```python
from build123d import *

# Parameters (mm, degrees)
SKETCH_5_R               = 3.5
EXTRUDE_2_DEPTH          = 13
SKETCH_6_R               = 3
CUT_EXTRUDE_2_DEPTH      = 13
CUT_EXTRUDE_2_DEPTH_BACK = 13
SKETCH_7_R               = 4.5
EXTRUDE_3_DEPTH          = 1.5


with BuildPart() as part:
    # Sketch 1 → Revolve 5 (revolve)
    with BuildSketch(Plane(origin=(0, 0, 0), x_dir=(1, 0, 0), z_dir=(0, 1, 0))):
        with BuildLine():
            Line((0, 5), (0, -5))
            ThreePointArc((0, -5), (-5, 0), (0, 5))
        make_face()
    revolve(axis=Axis((0, 0, -5), (0, 0, 1)))

    # Sketch 5 → Extrude 2 (add)
    with BuildSketch(Plane.XY):
        Circle(SKETCH_5_R)
    extrude(amount=EXTRUDE_2_DEPTH)

    # Sketch 6 → Cut-Extrude 2 (cut, two sides)
    with BuildSketch(Plane(origin=(0, 0, 0), x_dir=(0, 0, -1), z_dir=(1, 0, 0))) as cut_extrude_2_sk:
        Circle(SKETCH_6_R)
    extrude(amount=CUT_EXTRUDE_2_DEPTH, mode=Mode.SUBTRACT)
    extrude(cut_extrude_2_sk.sketch, amount=-CUT_EXTRUDE_2_DEPTH_BACK, mode=Mode.SUBTRACT)

    # Sketch 7 → Extrude 3 (add)
    with BuildSketch(Plane.XY.offset(5)):
        Circle(SKETCH_7_R)
    extrude(amount=-EXTRUDE_3_DEPTH)


solid = part.part
```
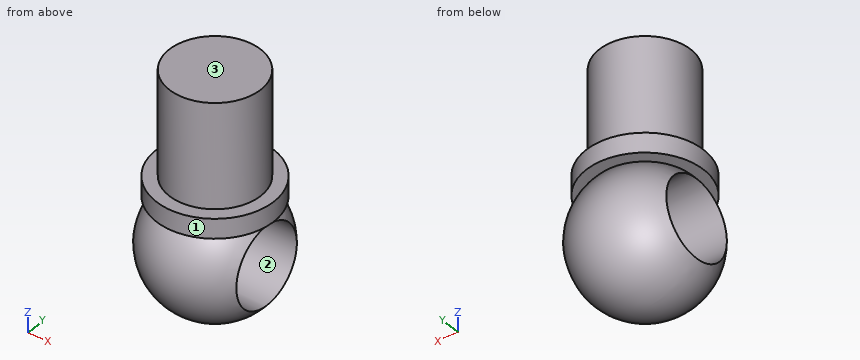
The listing builds one solid part. Answer for the finished solid, in the listing's coordinates (mm). Face numbers are marked on the shaded views. Round coordinates to 2 decimals unless told otherwise and drop trailing zeros. Write each loop counter-clockwise with the first axis right and the second up, starting at its lowest first coordinate (ties: lowest second). Pieces come first, ordered by that corner, then holes. Notation, with made-up numbers: (17, -5) -> (50, -5) arc R21 ccw to (50, 6) -> close; hole circle Ø6 at (46.5, 80.25). An arc over 180 degrees is marked (long way). Use CSV: the item, a comma, the result in double quotes. Start each with the question number.
(1) Section B-B on x = 0 is taken. Give the vertices of the cut face in (y, z).
(2) Section D-D on y = -2.75 is taken. Give the vertices of the cut face in (x, z), then the cut area to 3 significant figures.
(3) Section C-C on z = 0 is taken. Give the vertices of the cut face in (x, y).
(4) Each of these flat-tipped pins is pushed along its axis until it touches: pin 1 (6 mm diameter, centred on y = 4, z = 6, fed in from -X); pin 2 (5 mm diameter, centred on x = 2.5, y = 1, fed in from -Z); pin 3 (2 mm diameter, centred on x = -3, y = -2, fed in from -Z). Where does it stop, or does it pass through?
(5) Section A-A on y = -1.25 is taken. Give the vertices of the cut face in (x, z).
(6) The mould has two halves that part along Z. Classify the marked faces 1, 2 and 3: released by +Z, released by -Z, zero draft, split by the parting line, or undercut.
(7) Consider L1, parallel to Y at x = 0, z = 0; L2, parallel to Y at x = 0, z = 7; L3, parallel to Z at x = 0, y = -1.75. Determine where each line is inside the solid, lowest interval first. Write a range as from..to.
A:
1,outline,"(-4.5, 3.5) -> (-3.57, 3.5) arc R5 ccw (long way) to (3.57, 3.5) -> (4.5, 3.5) -> (4.5, 5) -> (3.5, 5) -> (3.5, 13) -> (-3.5, 13) -> (-3.5, 5) -> (-4.5, 5) -> close; hole circle Ø6 at (0, 0)"
2,outline,"(-4, -1.2) arc R4.18 ccw to (4, -1.2) -> close; (-4, 1.2) -> (4, 1.2) arc R4.18 ccw to (2.28, 3.5) -> (3.56, 3.5) -> (3.56, 5) -> (2.17, 5) -> (2.17, 13) -> (-2.17, 13) -> (-2.17, 5) -> (-3.56, 5) -> (-3.56, 3.5) -> (-2.28, 3.5) arc R4.18 ccw to start"
2,area,"78.3 mm²"
3,outline,"(-4, -3) arc R5 ccw to (4, -3) -> close; (-4, 3) -> (4, 3) arc R5 ccw to start"
4,pin 1,"stops at x = -4.34"
4,pin 2,"stops at z = -5"
4,pin 3,"stops at z = -4.27"
5,outline,"(-4.32, 3.5) -> (-3.34, 3.5) arc R4.84 ccw to (-4, 2.73) -> (4, 2.73) arc R4.84 ccw to (3.34, 3.5) -> (4.32, 3.5) -> (4.32, 5) -> (3.27, 5) -> (3.27, 13) -> (-3.27, 13) -> (-3.27, 5) -> (-4.32, 5) -> close; (-4, -2.73) arc R4.84 ccw to (4, -2.73) -> close"
6,face 1,"zero draft"
6,face 2,"undercut"
6,face 3,"released by +Z"
7,L1,"y = -5..-3, 3..5"
7,L2,"y = -3.5..3.5"
7,L3,"z = -4.68..-2.44, 2.44..13"
